Input: dimensioned drawing with shaded views. Units: mm. Origin: part minimum x, y, z. A direction names the side the tool comes from. Give positions to 0.01 mm unless a question says otherwise; leave off trailing zeros. Order: outer loops, then holes, each group sorted by start corner. A loop starts at its lowest first (then second) coordinate and runs counter-clockwise, first axis right, second up. Notation, with made-up numbers: (-26, 76) - (17, 76) arc R22 ccw to (17, 92) - close; hole circle Ø11 at (22.25, -30.5). An arc over 180 degrees is marked (long way). Answer as CSV lines item,"result".
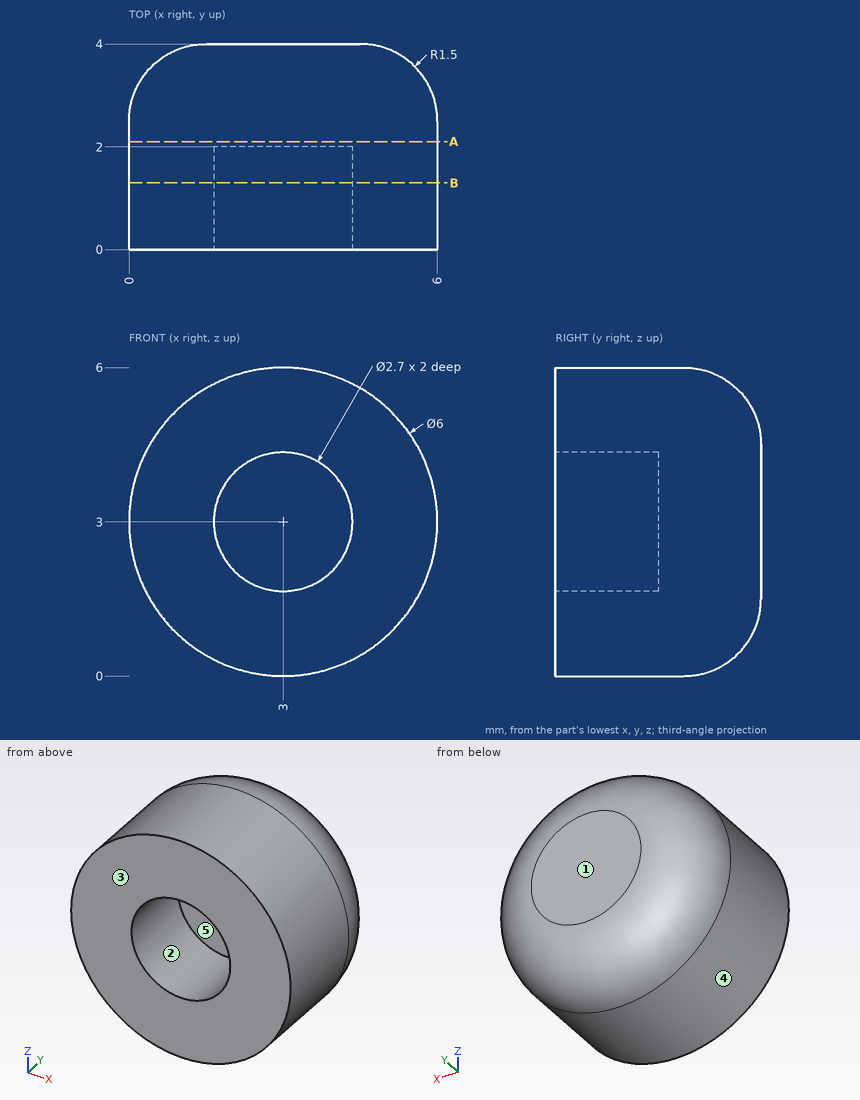
(1) Access query for the marked faces 1 and 2. Directions: +Z, -Z, +X, -X, +Y, -Y. A direction counts if a zero-diameter tool reaches every point of the face in a straight line with its end or side. Return the directions, or none.
Completed:
face 1,"+Z, -Z, +X, -X, +Y"
face 2,"-Y"
(2) Ray query, line 1 (Z direction, x = 3, y = 0.4); line 2 (Y direction, x = 3.9, z = 2.2); line 3 (X direction, y = 1.55, z = 2.55). Return the intervals inside material, ascending. Write a range as from..to.
Completed:
line 1,"0..1.65, 4.35..6"
line 2,"2..4"
line 3,"0.03..1.73, 4.27..5.97"
(3) Cut plane A-A (y = 2.1). Return loops of the section in (x, z), then the cut area to 3 significant figures.
Completed:
outline,"circle Ø6 at (3, 3)"
area,"28.3 mm²"
(4) Mould query, pull axis Z, two halves, no side actions, for the marked faces 3, 4 and 5. Classes: released by +Z, released by -Z, zero draft, split by the parting line, or undercut.
Completed:
face 3,"zero draft"
face 4,"split by the parting line"
face 5,"undercut"
(5) Contact query for a flat-ended pin moving along its axis: pin 1 (1.5 mm diameter, centred on y = 3.5, z = 2.5, fed in from -X). Output: stop coordinate, or through.
Completed:
pin 1,"x = 0.04"
(6) Cut plane B-B (y = 1.3). Return loops of the section in (x, z), then the cut area to 3 significant figures.
Completed:
outline,"circle Ø6 at (3, 3); hole circle Ø2.7 at (3, 3)"
area,"22.5 mm²"
